Answer from the drawing. Dimensions are ordinates in mm from the lowest x, y and z of the part. Round coordinates to 2 decimals unless told otherwise and drop trailing zeros. Write each loop counter-clockwise with the first axis right and the second up, starting at its lowest first coordinate (ties: lowest second). Pieces come first, ordered by that corner, then holes. Notation, with made-up numbers: (78.5, 20.25) -> (102.5, 20.25) arc R10 cw to (102.5, 26.25) -> close; hole circle Ø10 at (-36.5, 83.5). An arc over 180 degrees is marked (long way). Return JSON: item names as keys, results as strings. Group by question number.
(1) The mould has two halves that part along Y. Classify the marked faces 1, 2 and 3: released by +Y, released by -Y, zero draft, split by the parting line, or undercut.
(2) A cutting plane is placed at C-C on z = 16.25. Give the vertices of the cut face in (x, y).
(3) A cutting plane is placed at B-B on y = 17.25. Give the vertices of the cut face in (x, z) (1 decimal), then the cut area to 3 significant figures.
(4) A cutting plane is placed at D-D on y = 7.75. Give the vertices of the cut face in (x, z).
(5) A cutting plane is placed at A-A on z = 10.5. Give the vertices of the cut face in (x, y).
(6) Given pin 1 (3 mm diameter, centred on x = 2.5, y = 16, fed in from +Z), flat-ended and moving along its own axis, determine where the tip first touches the part or whether it passes through.
(7) Straight lines are drawn through the part: line 1 (Y direction, x = 5, z = 10.5); line 2 (X direction, y = 11.25, z = 1); line 3 (Z direction, x = 1.5, y = 10.5). For each, find the intervals that lie inside material, in ascending order.
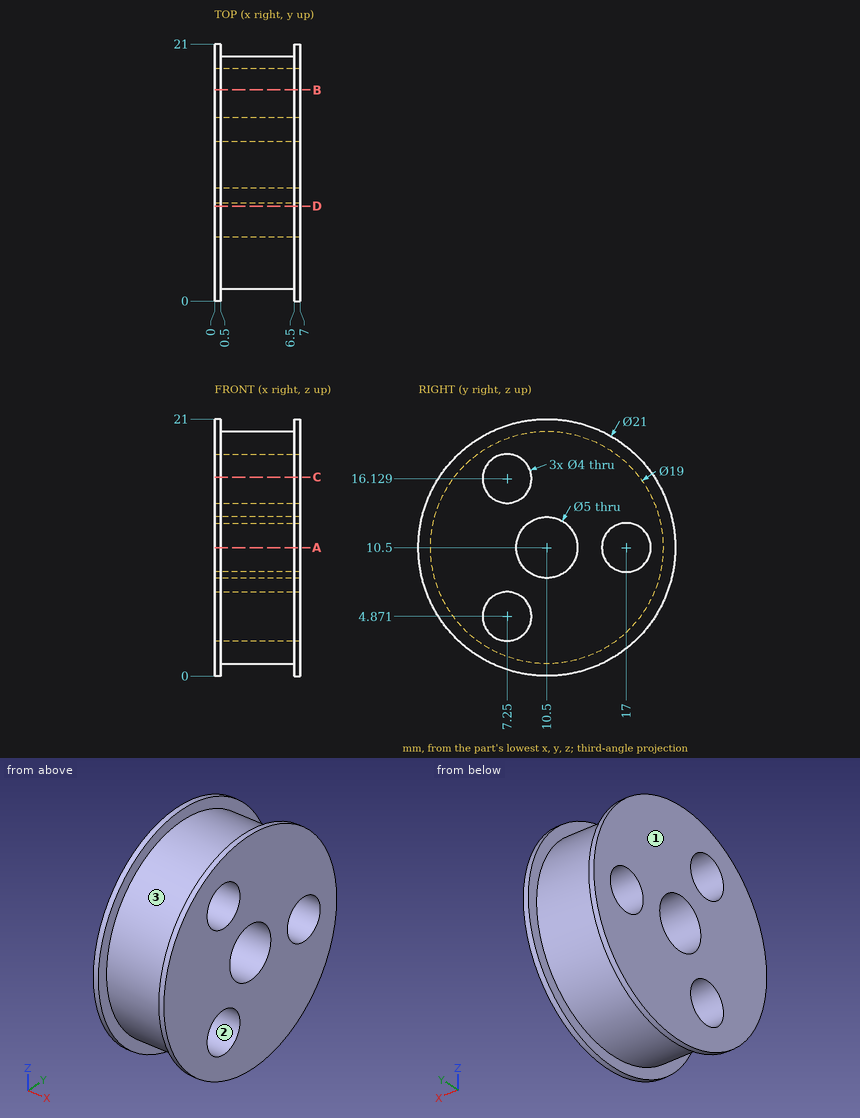
Checks:
{
 "1": {"face 1": "zero draft", "face 2": "undercut", "face 3": "split by the parting line"},
 "2": {"outline": "(0, 1.71) -> (0.5, 1.71) -> (0.5, 2.94) -> (6.5, 2.94) -> (6.5, 1.71) -> (7, 1.71) -> (7, 5.25) -> (0, 5.25) -> close; (0, 9.25) -> (7, 9.25) -> (7, 19.29) -> (6.5, 19.29) -> (6.5, 18.06) -> (0.5, 18.06) -> (0.5, 19.29) -> (0, 19.29) -> close"},
 "3": {"outline": "(0, 2.5) -> (0.5, 2.5) -> (0.5, 3.8) -> (6.5, 3.8) -> (6.5, 2.5) -> (7, 2.5) -> (7, 8.5) -> (0, 8.5) -> close; (0, 12.5) -> (7, 12.5) -> (7, 18.5) -> (6.5, 18.5) -> (6.5, 17.2) -> (0.5, 17.2) -> (0.5, 18.5) -> (0, 18.5) -> close", "area": "68.5 mm^2"},
 "4": {"outline": "(0, 0.37) -> (0.5, 0.37) -> (0.5, 1.41) -> (6.5, 1.41) -> (6.5, 0.37) -> (7, 0.37) -> (7, 2.93) -> (0, 2.93) -> close; (0, 6.81) -> (7, 6.81) -> (7, 14.19) -> (0, 14.19) -> close; (0, 18.07) -> (7, 18.07) -> (7, 20.63) -> (6.5, 20.63) -> (6.5, 19.59) -> (0.5, 19.59) -> (0.5, 20.63) -> (0, 20.63) -> close"},
 "5": {"outline": "(0, 0) -> (0.5, 0) -> (0.5, 1) -> (6.5, 1) -> (6.5, 0) -> (7, 0) -> (7, 8) -> (0, 8) -> close; (0, 13) -> (7, 13) -> (7, 15) -> (0, 15) -> close; (0, 19) -> (7, 19) -> (7, 21) -> (6.5, 21) -> (6.5, 20) -> (0.5, 20) -> (0.5, 21) -> (0, 21) -> close"},
 "6": {"pin 1": "stops at z = 19.12"},
 "7": {"line 1": "y = 1 to 8, 13 to 15, 19 to 20", "line 2": "x = 0 to 0.5, 6.5 to 7", "line 3": "z = 1 to 8, 13 to 20"}
}
